```python
from build123d import *

# Parameters (mm, degrees)
F0_R     = 50.8
F1_DEPTH = 25.4
F2_DEPTH = 25.4


with BuildPart() as f1:
    # F0 (on Top) → F1 (new body)
    with BuildSketch(Plane.XY):
        with Locations((-14.96590022, 9.497590363)):
            Circle(F0_R)
        with BuildLine():
            Line((-37.126943469, -16.1171220243), (-48.3513660729, -16.1171220243))
            Line((-48.3513660729, -16.1171220243), (-48.3513660729, 26.7659369856))
            Line((-48.3513660729, 26.7659369856), (-37.126943469, 26.7659369856))
            Line((-37.126943469, 26.7659369856), (-37.126943469, 23.0244621634))
            ThreePointArc((-37.126943469, 23.0244621634), (-25.562868863, 17.9519693026), (-25.6147123873, 5.3244074807))
            Line((-25.6147123873, 5.3244074807), (-14.96590022, 5.3244074807))
            Line((-14.96590022, 5.3244074807), (-14.96590022, 9.497590363))
            Line((-14.96590022, 9.497590363), (-14.96590022, 13.5268708691))
            Line((-14.96590022, 13.5268708691), (11.800034903, 13.5268708691))
            Line((11.800034903, 13.5268708691), (11.800034903, 16.9805400074))
            Line((11.800034903, 16.9805400074), (25.0390991569, 16.9805400074))
            Line((25.0390991569, 16.9805400074), (25.0390991569, -16.1171220243))
            Line((25.0390991569, -16.1171220243), (11.800034903, -16.1171220243))
            Line((11.800034903, -16.1171220243), (11.800034903, -2.8780577704))
            Line((11.800034903, -2.8780577704), (-37.126943469, -2.8780577704))
            Line((-37.126943469, -2.8780577704), (-37.126943469, -16.1171220243))
        make_face(mode=Mode.SUBTRACT)
    extrude(amount=F1_DEPTH)

    # F0 (on Top) → F2 (join)
    with BuildSketch(Plane.XY):
        with Locations((-14.96590022, 9.497590363)):
            Circle(F0_R)
        with BuildLine():
            Line((-37.126943469, -16.1171220243), (-48.3513660729, -16.1171220243))
            Line((-48.3513660729, -16.1171220243), (-48.3513660729, 26.7659369856))
            Line((-48.3513660729, 26.7659369856), (-37.126943469, 26.7659369856))
            Line((-37.126943469, 26.7659369856), (-37.126943469, 23.0244621634))
            ThreePointArc((-37.126943469, 23.0244621634), (-25.562868863, 17.9519693026), (-25.6147123873, 5.3244074807))
            Line((-25.6147123873, 5.3244074807), (-14.96590022, 5.3244074807))
            Line((-14.96590022, 5.3244074807), (-14.96590022, 9.497590363))
            Line((-14.96590022, 9.497590363), (-14.96590022, 13.5268708691))
            Line((-14.96590022, 13.5268708691), (11.800034903, 13.5268708691))
            Line((11.800034903, 13.5268708691), (11.800034903, 16.9805400074))
            Line((11.800034903, 16.9805400074), (25.0390991569, 16.9805400074))
            Line((25.0390991569, 16.9805400074), (25.0390991569, -16.1171220243))
            Line((25.0390991569, -16.1171220243), (11.800034903, -16.1171220243))
            Line((11.800034903, -16.1171220243), (11.800034903, -2.8780577704))
            Line((11.800034903, -2.8780577704), (-37.126943469, -2.8780577704))
            Line((-37.126943469, -2.8780577704), (-37.126943469, -16.1171220243))
        make_face(mode=Mode.SUBTRACT)
    extrude(amount=F2_DEPTH)


solid = f1.part
```
The listing builds one solid part. Answer for the finished solid, in the listing's coordinates (mm). A direction names the side the tool comes from. Round coordinates to 2 decimals unless told otherwise and drop trailing zeros. Loops run counter-clockwise (first coordinate to the right, second up) from the corner with the lowest first, then second, coordinate; pieces in that order, holes last. Notation, with made-up numbers: (47, 15) - (79, 15) arc R21 cw to (79, 21) - close; hole circle Ø4 at (67.25, -7). An arc over 180 degrees is marked (long way). Use one line per item in the form item = value. Start each with the question number.
1. The part is cut by section B-B on y = 21.5. Determine the outline of the cut face in (x, z).
2. A tool of negligible diameter and unlimited length cuts with its end or side. For faces 4 (the face through (-16, 10, 25.4)), 5 (the face through (-37.127, -9, 13)), from which of +Z, -Z, +X, -X, +Y, -Y can it reach the whole face along a straight path? Write none if from no direction.
3. The part is cut by section C-C on z = 23. Determine the outline of the cut face in (x, y).
4. The part is cut by section D-D on y = -20.5. Determine the outline of the cut face in (x, z), then the cut area to 3 significant figures.
5. Given pin 1 Ø14.5 at (x, z) = (18, 18) entering from +Y; pin 2 Ø2 at (x, y) = (5.5, -10) entering from -Z; pin 3 Ø1.5 at (x, z) = (-19, 7.5) entering from +Y; pin 4 Ø1.5 at (y, z) = (-25, 12) entering from +X, each flat-ended and moving along its own axis, determine where each tip first touches the part or whether it passes through.
6. For a pull along X with two mould halves and no side action, classify faces 1 (the face through (-43, -16.117, 13)), 2 (the face through (-16, 10, 0)), 3 (the face through (-65.717, 11.731, 12.522)) as pulls with the +X half, pulls with the -X half, needs draft (parallel to the pull), parting line crosses it, or undercut.
7. The part is cut by section A-A on x = -30. Determine the outline of the cut face in (y, z).
8. Consider line 1 (X direction, y = -7.5, z = 16.75); line 2 (X direction, y = -9.5, z = 7.5); line 3 (Y direction, x = 14, z = 5.5). Determine where each line is inside the solid, lowest interval first. Write a range as [from, to].
Geometry check:
q1.outline = (-64.33, 0) - (-48.35, 0) - (-48.35, 25.4) - (-64.33, 25.4) - close; (-29.21, 0) - (34.4, 0) - (34.4, 25.4) - (-29.21, 25.4) - close
q2.face_4 = +Z, +X, -X, +Y, -Y
q2.face_5 = +Z, -Z
q3.outline = circle Ø101.6 at (-14.97, 9.5); hole (-48.35, -16.12) - (-37.13, -16.12) - (-37.13, -2.88) - (11.8, -2.88) - (11.8, -16.12) - (25.04, -16.12) - (25.04, 16.98) - (11.8, 16.98) - (11.8, 13.53) - (-14.97, 13.53) - (-14.97, 5.32) - (-25.61, 5.32) arc R11.51 ccw to (-37.13, 23.02) - (-37.13, 26.77) - (-48.35, 26.77) - close
q4.outline = (-55.96, 0) - (26.03, 0) - (26.03, 25.4) - (-55.96, 25.4) - close
q4.area = 2,080 mm^2
q5.pin_1 = 53.31
q5.pin_2 = 0
q5.pin_3 = 60.19
q5.pin_4 = 23
q6.face_1 = undercut
q6.face_2 = needs draft
q6.face_3 = parting line crosses it
q7.outline = (-39.03, 0) - (-2.88, 0) - (-2.88, 25.4) - (-39.03, 25.4) - close; (21.94, 0) - (58.02, 0) - (58.02, 25.4) - (21.94, 25.4) - close
q8.line_1 = [-62.84, -48.35], [-37.13, 11.8], [25.04, 32.91]
q8.line_2 = [-62.08, -48.35], [-37.13, 11.8], [25.04, 32.15]
q8.line_3 = [-32.24, -16.12], [16.98, 51.23]
